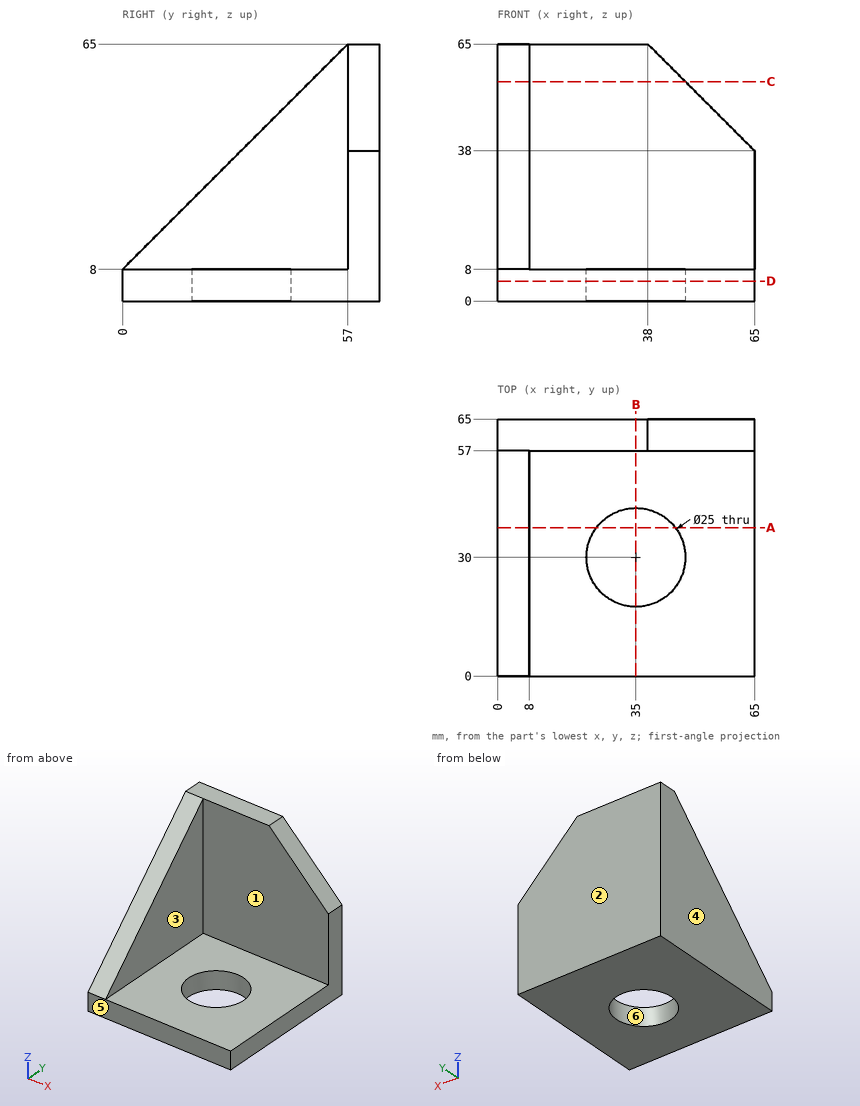
Geometry check sheet. Reference: drawing and pictorial views, mm from the part's lowest x, y, z. A direction names the side the tool comes from. Give positions to 0.01 mm unless a question says otherwise; leave off trailing zeros. Order: outer loops, then holes, each group sorted by start corner. A loop starts at its lowest first (then second) coordinate and runs counter-clockwise, first axis right, second up. Notation, with made-up numbers: M -10.75,47.25 L 16.25,47.25 A20 ccw 16.25,54.25 Z; hole C 13.5,-37.75 d9. An arc over 180 degrees is marked long. Answer in a Markdown table with one row per item.
1) Cross-section at D-D, the plane z = 5. Enter the section's corners in (x, y).
Filled sheet:
| item | result |
|---|---|
| outline | M 0,0 L 65,0 L 65,65 L 0,65 Z; hole C 35,30 d25 |
2) Release check for a two-part mould opening along X. For the marked faces 3, 4, 5 and 6 record: +X half, -X half, draft (parallel to the pull), parting line (faces both ways), or undercut.
Filled sheet:
| item | result |
|---|---|
| face 3 | +X half |
| face 4 | -X half |
| face 5 | draft |
| face 6 | undercut |
3) Cross-section at B-B, the plane x = 35. Enter the section's corners in (y, z).
Filled sheet:
| item | result |
|---|---|
| outline | M 0,0 L 17.5,0 L 17.5,8 L 0,8 Z; M 42.5,0 L 65,0 L 65,65 L 57,65 L 57,8 L 42.5,8 Z |
4) Gauge pin test, flat ends, axial feed: P1, Ø4, axis at x = 36, z = 31, coming from the -Y side; P2, Ø17, axis at x = 27.5, y = 37.5, coming from the +Z side; P3, Ø22.5, axis at x = 35, y = 30, coming from the +Z side. Record the tip position at first contact, or that the pin passes through.
Filled sheet:
| item | result |
|---|---|
| P1 | stops at y = 57 |
| P2 | stops at z = 8 |
| P3 | passes through |
5) Access from +Z, -Z, +X, -X, +Y, -Y to the whole of each face (thin tool, end or side, straight path). Record for the marked faces 1 and 2.
Filled sheet:
| item | result |
|---|---|
| face 1 | +Z, +X, -Y |
| face 2 | +Z, -Z, +X, -X, +Y |
6) Thickness scan on L1, parallel to Y at x = 35, z = 5; L2, parallel to Z at x = 17.5, y = 12.5; L3, parallel to Y at x = 31.5, z = 3.5. Record the ranges inside material, lowest first. Write a range as [from, to].
Filled sheet:
| item | result |
|---|---|
| L1 | y = [0, 17.5], [42.5, 65] |
| L2 | z = [0, 8] |
| L3 | y = [0, 18], [42, 65] |
7) Cross-section at A-A, the plane y = 37.5. Enter the section's corners in (x, z), plus the area to 3 significant figures.
Filled sheet:
| item | result |
|---|---|
| outline | M 0,0 L 25,0 L 25,8 L 8,8 L 8,45.5 L 0,45.5 Z; M 45,0 L 65,0 L 65,8 L 45,8 Z |
| area | 660 mm2 |
8) Cross-section at C-C, the plane z = 55.5. Enter the section's corners in (x, y), plus the area to 3 significant figures.
Filled sheet:
| item | result |
|---|---|
| outline | M 0,47.5 L 8,47.5 L 8,57 L 47.5,57 L 47.5,65 L 0,65 Z |
| area | 456 mm2 |
